Input: part model. Units: mm. Frame: model coordinates. A direction names the side the tool comes from. Round coordinates to 2 decimals unless told otherwise and drop trailing zeros. Loops run counter-clockwise (first coordinate to the right, second up) from the corner with the lowest first, then second, coordinate; pieces in that order, holes last. Notation, with made-up numbers: (13.25, 23) - (41.25, 23) arc R33 ccw to (41.25, 61) - close; hole circle Ø11 at (71, 7.25). An arc over 180 degrees is marked (long way). One line per question, with ' | ' between items. Start each with the question number.
Item 1: First-contact query: pin 1 (1.3 mm diameter, centred on x = -1.5, y = -34.5, fed in from +Z); pin 2 (4 mm diameter, centred on x = 3, y = -15.5, fed in from -Z); pin 3 (1.3 mm diameter, centred on x = 13, y = 8.5, fed in from +Z); pin 4 (0.7 mm diameter, centred on x = -9, y = -4.5, fed in from +Z). Flat tips, straight axial feed; report the tip coordinate or a pass-through.
Item 2: Section D-D, the plane x = 0.5. Give the number of separate pieces and of enclosed holes in the cut face, plus the area to 3 significant figures.
Item 3: Section C-C, the plane z = 13. Return loops of the section in (x, y).
Item 4: Section A-A, the plane z = 20. Return loops of the section in (x, y).
Item 5: Draft query along Z for faces 6 (the face through (-13.4, 4.9, 7.5)), 7 (the face through (3.649, -9.123, 5.944)), 8 (the face through (2.7, 0.5, 2)). Return one class per face: pulls with the +Z half, pulls with the -Z half, needs draft (parallel to the pull), parting line crosses it, or undercut.
Item 6: Material intervals for line 1 along Y through (x, z) = (9, 10.25); line 2 along X through (y, z) = (-18, 21.25); line 3 along Z through (x, y) = (-13.55, 6.5), sorted ascending.
Item 7: Section B-B, the plane y = 6.5. Return loops of the section in (x, z).
Item 8: Set-up query: faces 1 (the face through (-5.508, -12.956, 4.93)), 2 (the face through (-13.5, 18.3, 23)), 3 (the face through (0, -34, 15.8)), 4 (the face through (13, 20.8, 20)), 5 (the face through (3.815, 17.401, 5.944)). Return all of +Z, -Z, +X, -X, +Y, -Y with unobstructed straight access to the full face (end or side cutting, diameter ignored); none if empty.
```python
from build123d import *

# Parameters (mm, degrees)
SKETCH_W        = 28
SKETCH_H        = 70
PAD_DEPTH       = 23
SKETCH001_W     = 25.6
SKETCH001_H     = 67.6
POCKET_DEPTH    = 21
SKETCH002_W     = 1.2
SKETCH002_H     = 33
POCKET001_DEPTH = 5.5
SKETCH003_R     = 2.6
SKETCH003_R_2   = 1.1
PAD001_DEPTH    = 15
SKETCH004_R     = 3.1
SKETCH004_R_2   = 1.9
POCKET002_DEPTH = 2
SKETCH005_R     = 4
SKETCH005_R_2   = 3.1
SKETCH005_R_3   = 2.7
SKETCH005_R_4   = 1.9
PAD002_DEPTH    = 8
SKETCH006_W     = 8.4
SKETCH006_H     = 1.2
POCKET003_DEPTH = 7.2
SKETCH007_R     = 3.4
POCKET004_DEPTH = 2
FILLET_R        = 1


with BuildPart() as part:
    # Sketch → Pad (new body)
    with BuildSketch(Plane.XY):
        Rectangle(SKETCH_W, SKETCH_H)
    extrude(amount=PAD_DEPTH)

    # Sketch001 → Pocket (cut)
    with BuildSketch(Plane.XY.offset(23)):
        Rectangle(SKETCH001_W, SKETCH001_H)
    extrude(amount=-POCKET_DEPTH, mode=Mode.SUBTRACT)

    # Sketch002 → Pocket001 (cut)
    with BuildSketch(Plane.XY.offset(23)):
        with Locations((13.4, 4.3)):
            Rectangle(SKETCH002_W, SKETCH002_H)
    extrude(amount=-POCKET001_DEPTH, mode=Mode.SUBTRACT)

    # Sketch003 → Pad001 (new body)
    with BuildSketch(Plane.XY.offset(2)):
        with Locations((-9, -3.8)):
            Circle(SKETCH003_R)
        with Locations((-9, -3.8)):
            Circle(SKETCH003_R_2, mode=Mode.SUBTRACT)
        with Locations((-9, 27.2)):
            Circle(SKETCH003_R)
        with Locations((-9, 27.2)):
            Circle(SKETCH003_R_2, mode=Mode.SUBTRACT)
        with Locations((9, 27.2)):
            Circle(SKETCH003_R)
        with Locations((9, 27.2)):
            Circle(SKETCH003_R_2, mode=Mode.SUBTRACT)
    extrude(amount=PAD001_DEPTH)

    # Sketch004 → Pocket002 (cut)
    with BuildSketch(Plane.XY.offset(2)):
        with Locations((0, 25.2)):
            Circle(SKETCH004_R)
        with Locations((0, 16.2)):
            Circle(SKETCH004_R)
        with Locations((0, -2.8)):
            Circle(SKETCH004_R)
        with Locations((-4, -11.8)):
            Circle(SKETCH004_R_2)
        with Locations((4, -11.8)):
            Circle(SKETCH004_R_2)
    extrude(amount=-POCKET002_DEPTH, mode=Mode.SUBTRACT)

    # Sketch005 → Pad002 (new body)
    with BuildSketch(Plane.XY.offset(2)):
        with Locations((0, 25.2)):
            Circle(SKETCH005_R)
        with Locations((0, 25.2)):
            Circle(SKETCH005_R_2, mode=Mode.SUBTRACT)
        with Locations((0, 16.2)):
            Circle(SKETCH005_R)
        with Locations((0, 16.2)):
            Circle(SKETCH005_R_2, mode=Mode.SUBTRACT)
        with Locations((0, -2.8)):
            Circle(SKETCH005_R)
        with Locations((0, -2.8)):
            Circle(SKETCH005_R_2, mode=Mode.SUBTRACT)
        with Locations((-4, -11.8)):
            Circle(SKETCH005_R_3)
        with Locations((-4, -11.8)):
            Circle(SKETCH005_R_4, mode=Mode.SUBTRACT)
        with Locations((4, -11.8)):
            Circle(SKETCH005_R_3)
        with Locations((4, -11.8)):
            Circle(SKETCH005_R_4, mode=Mode.SUBTRACT)
    extrude(amount=PAD002_DEPTH)

    # Sketch006 → Pocket003 (cut)
    with BuildSketch(Plane.XY.offset(23)):
        with Locations((0, -34.4)):
            Rectangle(SKETCH006_W, SKETCH006_H)
    extrude(amount=-POCKET003_DEPTH, mode=Mode.SUBTRACT)

    # Sketch007 → Pocket004 (cut)
    with BuildSketch(Plane(origin=(-14, 0, 0), x_dir=(0, -1, 0), z_dir=(-1, 0, 0))):
        with Locations((-6.5, 10.5)):
            Circle(SKETCH007_R)
    extrude(amount=-POCKET004_DEPTH, mode=Mode.SUBTRACT)

    # Fillet
    fillet_edges = [part.edges().sort_by_distance(p)[0] for p in [
        (-14, 35, 11.5),
        (-14, -35, 11.5),
        (14, -35, 11.5),
        (14, 35, 11.5),
    ]]
    fillet(fillet_edges, radius=FILLET_R)


solid = part.part
```
Return value:
1) pin 1: z = 15.8 | pin 2: z = 0 | pin 3: z = 17.5 | pin 4: z = 2
2) separate pieces: 4 | enclosed holes: 0 | area: 189 mm2
3) outline: (-14, -34) arc R1 ccw to (-13, -35) - (13, -35) arc R1 ccw to (14, -34) - (14, 34) arc R1 ccw to (13, 35) - (-13, 35) arc R1 ccw to (-14, 34) - (-14, 8.8) - (-12.8, 8.8) - (-12.8, 33.8) - (12.8, 33.8) - (12.8, -33.8) - (-12.8, -33.8) - (-12.8, 4.2) - (-14, 4.2) - close; circle Ø5.2 at (-9, -3.8); circle Ø5.2 at (-9, 27.2); circle Ø5.2 at (9, 27.2); hole circle Ø2.2 at (-9, -3.8); hole circle Ø2.2 at (-9, 27.2); hole circle Ø2.2 at (9, 27.2)
4) outline: (-14, -34) arc R1 ccw to (-13, -35) - (-4.2, -35) - (-4.2, -33.8) - (-12.8, -33.8) - (-12.8, 33.8) - (12.8, 33.8) - (12.8, 20.8) - (14, 20.8) - (14, 34) arc R1 ccw to (13, 35) - (-13, 35) arc R1 ccw to (-14, 34) - close; (4.2, -35) - (13, -35) arc R1 ccw to (14, -34) - (14, -12.2) - (12.8, -12.2) - (12.8, -33.8) - (4.2, -33.8) - close
5) face 6: undercut | face 7: needs draft | face 8: pulls with the +Z half
6) line 1: -35 to -33.8, 24.6 to 26.1, 28.3 to 29.8, 33.8 to 35 | line 2: -14 to -12.8, 12.8 to 14 | line 3: 0 to 7.1, 13.9 to 23
7) outline: (-14, 0) - (14, 0) - (14, 17.5) - (12.8, 17.5) - (12.8, 2) - (-12.8, 2) - (-12.8, 7.1) - (-14, 7.1) - close; (-14, 13.9) - (-12.8, 13.9) - (-12.8, 23) - (-14, 23) - close
8) face 1: +Z, -Z | face 2: +Z, +X, -X, +Y, -Y | face 3: +Z, -Y | face 4: +Z, +X | face 5: +Z
